from build123d import *

# Parameters (mm, degrees)
SKETCH1_W          = 25.4
SKETCH1_H          = 120.65
EXTRUDE1_DEPTH     = 444.5
SKETCH2_R          = 25.4
CUT_EXTRUDE1_DEPTH = 25.4
CUT_EXTRUDE2_DEPTH = 50.8


with BuildPart() as part:
    # Sketch1 → Extrude1 (new body)
    with BuildSketch(Plane.XY):
        with Locations((0, 60.325)):
            Rectangle(SKETCH1_W, SKETCH1_H)
    extrude(amount=-EXTRUDE1_DEPTH)

    # Sketch2 → Cut-Extrude1 (cut, symmetric)
    with BuildSketch(Plane(origin=(0, 0, 0), x_dir=(0, 0, -1), z_dir=(1, 0, 0))):
        with Locations((382.5748, 49.2252)):
            Circle(SKETCH2_R)
    extrude(amount=CUT_EXTRUDE1_DEPTH, both=True, mode=Mode.SUBTRACT)

    # Sketch4 → Cut-Extrude2 (cut)
    with BuildSketch(Plane(origin=(0, 0, -369.8748), x_dir=(-1, 0, 0), z_dir=(0, 0, -1))):
        Polygon((-22.207602217, 34.907602217), (28.73114164, -16.03114164), (-22.207602217, -16.03114164), align=None)
    extrude(amount=-CUT_EXTRUDE2_DEPTH, mode=Mode.SUBTRACT)


solid = part.part
Here's how the part is built. I have some questions about the finished solid (model axes, mm). A direction names the side the tool comes from. Round coordinates to 2 decimals unless told otherwise and drop trailing zeros. Loops run counter-clockwise (first coordinate to the right, second up) from the corner with the lowest first, then second, coordinate; pieces in that order, holes last. Notation, with made-up numbers: M 47,57 L 78,57 A29 cw 78,82 Z; hole C -38,33.5 d2. An arc over 180 degrees is marked long. Write each question's results on one line, items separated by ' | '. Start each with the question number.
(1) I want a section at A-A (y = 8). Please give me the cut outline in (x, z).
(2) On a 3-axis mill with a long thin cutter (end or side, diameter ignored), from which of +Z, -Z, +X, -X, +Y, -Y can I reach the whole of each face in a straight line? I mean faces 4 (the flat face through (5, 7, -319.075)), 5 (the cylindrical face through (0.18, 50.34, -357.2)). Say none if no direction works.
(3) If I drill on probe 1 along Z at (x, y) = (10.5, 48); probe 2 along Z at (x, y) = (8, 35.5); probe 3 along Y at (x, z) = (9, -378), over which ranges is the centre line in solid material (lowest first)? Write a range as from..to.
(4) Will these pins go through, and if not, where does the flat tip stop? P1, Ø3, axis at x = -8.5, z = -344.5, coming from the -Y side; P2, Ø1.5, axis at x = -4, y = 70, coming from the +Z side.
(5) I want a section at D-D (y = 33). Please give me the cut outline in (x, z), then the cut area to 3 significant figures.
(6) Thinking about a two-plate mould opening in Z: for faces 1 (the flat face through (0, 61, -444.5)), 2 (the flat face through (5, 7, -369.875)), 3 (the flat face through (0, 0, -157)), which applies, pulls with the +Z half, pulls with the -Z half, needs draft (parallel to the pull), parting line crosses it, or undercut?
(7) I want a section at B-B (x = -4.25). Please give me the cut outline in (y, z), then the cut area to 3 significant figures.
(8) I want a section at C-C (y = 56.5). Please give me the cut outline in (x, z).
Solved:
1) outline: M -12.7,-444.5 L 12.7,-444.5 L 12.7,-369.87 L -4.7,-369.87 L -4.7,-319.07 L 12.7,-319.07 L 12.7,0 L -12.7,0 Z
2) face 4: +X, -Y | face 5: +X, -X
3) probe 1: z = -444.5..-407.95, -357.2..0 | probe 2: z = -444.5..-403.95, -361.2..0 | probe 3: y = 0..24.24, 74.21..120.65
4) P1: stops at y = 2.7 | P2: stops at z = 0
5) outline: M -12.7,-444.5 L 12.7,-444.5 L 12.7,-402.12 L -12.7,-402.12 Z; M -12.7,-363.03 L 12.7,-363.03 L 12.7,0 L -12.7,0 Z | area: 10,300 mm²
6) face 1: pulls with the -Z half | face 2: undercut | face 3: needs draft
7) outline: M 0,-444.5 L 120.65,-444.5 L 120.65,0 L 0,0 L 0,-319.07 L 8.45,-319.07 L 8.45,-369.87 L 0,-369.87 Z; hole C 49.23,-382.57 d50.8 | area: 51,200 mm²
8) outline: M -12.7,-444.5 L 12.7,-444.5 L 12.7,-406.91 L -12.7,-406.91 Z; M -12.7,-358.24 L 12.7,-358.24 L 12.7,0 L -12.7,0 Z
